Can you work these out from the model? Positions are in its coordinate system, mm. A direction names the side the tool comes from. Round coordinates to 2 decimals unless told otherwise and drop trailing zeros. Loops run counter-clockwise (first coordinate to the right, second up) from the corner with the lowest first, then second, coordinate; pieces in that order, holes last. Notation, with made-up numbers: M 59,-25.5 L 112,-25.5 A20 cw 112,-13.5 Z; hole C 38.25,33.25 d5. An arc over 180 degrees is marked long. Return JSON: item names as keys, results as strings.
Autodesk Inventor part; units mm, degrees
ref_plane "YZ Plane" through (0, 0, 0) normal (1, 0, 0) x (0, 1, 0)
ref_plane "XZ Plane" through (0, 0, 0) normal (0, 1, 0) x (-1, 0, 0)
ref_plane "XY Plane" through (0, 0, 0) normal (0, 0, 1) x (1, 0, 0)
sketch "Sketch2" plane through (0, 0, 0) normal (0, 1, 0) x (-1, 0, 0)
  line L0 (90, 130) -> (-90, -130) construction
  line L1 (-90, 130) -> (90, -130) construction
  circle A0 centre (65, 105) radius 10
  circle A1 centre (-65, 105) radius 10
  circle A2 centre (-65, -105) radius 10
  circle A3 centre (65, -105) radius 10
  line L2 (0, 65.8121) -> (0, -50.2865) construction
  line L3 (90, 0) -> (70, 0) construction
  line L4 (90, -8) -> (70, -8)
  line L5 (70, 8) -> (90, 8)
  arc A4 (70, 8) -> (70, -8) centre (70, 0) ccw
  line L6 (-90, -8) -> (-70, -8)
  line L7 (-70, 8) -> (-90, 8)
  arc A5 (-70, -8) -> (-70, 8) centre (-70, 0) ccw
  line L8 (90, -130) -> (90, -8)
  line L9 (90, 8) -> (90, 130)
  line L10 (-90, 130) -> (-90, 8)
  line L11 (-90, -8) -> (-90, -130)
  line L12 (0, -110) -> (0, -154.4719) construction
  line L13 (-8, -110) -> (-8, -130)
  line L14 (8, -130) -> (8, -110)
  arc A6 (8, -110) -> (-8, -110) centre (0, -110) ccw
  line L15 (25.1981, 0) -> (-33.3058, 0) construction
  line L16 (-8, 110) -> (-8, 130)
  line L17 (8, 130) -> (8, 110)
  arc A7 (-8, 110) -> (8, 110) centre (0, 110) ccw
  line L18 (90, 130) -> (8, 130)
  line L19 (-8, 130) -> (-90, 130)
  line L20 (-90, -130) -> (-8, -130)
  line L21 (8, -130) -> (90, -130)
  point P0 (0, 0)
  point P1 (80, 0)
  point P2 (0, -132.2359)
  point P3 (8, 154.4719)
  dimension "d2" = 180
  dimension "d3" = 260
  dimension "d4" = 20
  dimension "d6" = 65
  dimension "d7" = 65
  dimension "d9" = 65
  dimension "d12" = 65
  dimension "d16" = 8
  dimension "d18" = 8
  dimension "d33" = 180
  dimension "d34" = 260
extrude "Extrusion2" add sketch "Sketch2" along normal blind 20
sketch "Sketch3" plane through (0, 20, 0) normal (0, 1, 0) x (1, 0, 0)
  circle A0 centre (0, 35) radius 2.5
  circle A1 centre (-35, 0) radius 2.5
  circle A2 centre (0, -35) radius 2.5
  circle A3 centre (35, 0) radius 2.5
  point P0 (0, 0)
  dimension "d22" = 5
  dimension "d23" = 35
  dimension "d26" = 360
extrude "Extrusion3" cut sketch "Sketch3" against normal blind 12
sketch "Sketch4" plane through (0, 20, 0) normal (0, 1, 0) x (1, 0, 0)
  circle A0 centre (0, 0) radius 20
  dimension "d30" = 40
extrude "Extrusion4" cut sketch "Sketch4" against normal blind 10
properties part number "Base inferior da ferramenta"
Q1. Suppose I cut it at A-A, the plane y = 15.75. State how many separate pieces and enclosed holes the cut face has, plus the area to 3 significant figures.
Results:
{"separate pieces": "1", "enclosed holes": "9", "area": "42,500 mm2"}
Q2. I'm going to push flat-ended pins straight in: pin 1 Ø1 at (x, z) = (65.5, 96.5) entering from +Y; pin 2 Ø1.5 at (x, z) = (1, -35) entering from +Y. Where does each tip first touch, or does it pass through?
Results:
{"pin 1": "passes through", "pin 2": "stops at y = 8"}
Q3. Thinking about a two-plate mould opening in Z: for faces 1 (the flat face through (90, 10, 70)), 2 (the flat face through (-50, 10, 130)), 3 (the cylindrical face through (-62, 10, 0)), 4 (the cylindrical face through (-57.63, 9.86, -111.76)), which applies, pulls with the +Z half, pulls with the -Z half, needs draft (parallel to the pull), parting line crosses it, or undercut?
Results:
{"face 1": "needs draft", "face 2": "pulls with the +Z half", "face 3": "undercut", "face 4": "undercut"}
Q4. Suppose I cut it at B-B, the plane x = 65. Please give me the cut outline in (y, z) (3 decimals), plus the area to 3 significant figures.
Results:
{"outline": "M 0,-130 L 20,-130 L 20,-115 L 0,-115 Z; M 0,-95 L 20,-95 L 20,-6.245 L 0,-6.245 Z; M 0,6.245 L 20,6.245 L 20,95 L 0,95 Z; M 0,115 L 20,115 L 20,130 L 0,130 Z", "area": "4,150 mm2"}
Q5. On a 3-axis mill with a long thin cutter (end or side, diameter ignored), from which of +Z, -Z, +X, -X, +Y, -Y can I reach the whole of each face in a straight line? I mean faces 5 (the flat face through (-80, 10, -8)), 6 (the flat face through (-8, 10, 120)), 7 (the cylindrical face through (1.34, 14.08, 32.89)), 8 (the flat face through (80, 10, -8)), 9 (the flat face through (-8, 10, -120)). Say none if no direction works.
Results:
{"face 5": "-X, +Y, -Y", "face 6": "+Z, +Y, -Y", "face 7": "+Y", "face 8": "+X, +Y, -Y", "face 9": "-Z, +Y, -Y"}
Q6. If I drill on line 1 along X through (y, z) = (18.25, 0); line 2 along Z through (x, y) = (35, 17); line 3 along X through (y, z) = (10, 110), over which ranges is the centre line in solid material (lowest first)?
Results:
{"line 1": "x = -62 to -37.5, -32.5 to -20, 20 to 32.5, 37.5 to 62", "line 2": "z = -130 to -2.5, 2.5 to 130", "line 3": "x = -90 to -73.66, -56.34 to -8, 8 to 56.34, 73.66 to 90"}
